Autodesk Inventor part; units mm, degrees
ref_plane "YZ Plane" through (0, 0, 0) normal (1, 0, 0) x (0, 1, 0)
ref_plane "XZ Plane" through (0, 0, 0) normal (0, 1, 0) x (-1, 0, 0)
ref_plane "XY Plane" through (0, 0, 0) normal (0, 0, 1) x (1, 0, 0)
sketch "Sketch1" plane through (0, 0, 0) normal (1, 0, 0) x (0, 1, 0)
  line L0 (0, 0) -> (12.7, 0)
  line L1 (12.7, 0) -> (12.7, -25.4)
  line L2 (12.7, -25.4) -> (0, -25.4)
  line L3 (0, -25.4) -> (0, 0)
  dimension "d0" = 12.7
  dimension "d1" = 25.4
extrude "Extrusion1" add sketch "Sketch1" along normal blind 4.7752
sketch "Sketch2" plane through (0, 12.7, 0) normal (0, 1, 0) x (1, 0, 0)
  line L0 (0, 25.4) -> (4.7752, 25.4)
  line L1 (0, 0) -> (4.7752, 0)
  point P0 (2.2104, 5.08)
  point P1 (2.2104, 20.32)
  dimension "d22" = 5.08
  dimension "d23" = 5.08
hole "Hole1" at (2.2104, 12.7, -5.08) at (2.2104, 12.7, -20.32) direction (0, -1, 0) diameter 3.429 end through all
sketch "Sketch3" plane through (0, 0, 0) normal (-1, 0, 0) x (0, 0, 1)
  line L0 (0, 12.7) -> (-25.4, 12.7)
  line L1 (-25.4, 0) -> (0, 0)
  line L2 (0, 0) -> (0, 12.7)
  point P0 (-12.7, 6.35)
  dimension "d11" = 12.7
  dimension "d12" = 25.4
  dimension "d13" = 6.35
  dimension "d14" = 12.7
hole "Hole2" at (0, 6.35, -12.7) direction (1, 0, 0) diameter 3.429 end through all
properties part number "WheelIntakeSpringStop"
Design review of the part built by this model. Coordinates are the model's own, in mm. Give positions to 0.01 mm unless a question says otherwise; leave off trailing zeros. Write each loop counter-clockwise with the first axis right and the second up, starting at its lowest first coordinate (ties: lowest second). Pieces come first, ordered by that corner, then holes. Notation, with made-up numbers: M -26,87 L -22,87 A18 ccw -22,103 Z; hole C -15,78.25 d5. An arc over 180 degrees is marked long. Answer as a JSON object with one key per item and string values. Group by question number.
1) We need section C-C (y = 11.75). Give the boundary of the cut face in (x, z), and give its area (3 significant figures).
2) We need section B-B (z = -12.7). Give the boundary of the cut face in (x, y).
3) For line 1 along Z through (x, y) = (2.1, 10); line 2 along Z through (x, y) = (2.35, 6.35); line 3 along X through (y, z) = (8, -20.32), list the stretches that pass through material, from the lowest coordinate up.
4) Clearance check with flat-ended pins moving along their axes: pin 1 Ø2.5 at (y, z) = (6.35, -12.7) entering from +X; pin 2 Ø1.5 at (x, y) = (1, 1.5) entering from +Z. State where each tip first meets the part, or that it passes through.
5) We need section A-A (y = 6.35). Give the boundary of the cut face in (x, z), and give its area (3 significant figures).
6) We need section D-D (z = -20.32). Give the boundary of the cut face in (x, y).
7) Mouldability with a two-part tool opening along Z and no side actions: class faces 1 (the face through (2, 12.7, -13)), 2 (the face through (2.421, 5.835, -11.065)), 3 (the face through (2, 6, -25.4)) as released by +Z, released by -Z, zero draft, split by the parting line, or undercut.
Answer key:
{
 "1": {"outline": "M 0,-25.4 L 4.78,-25.4 L 4.78,0 L 0,0 Z; hole C 2.21,-20.32 d3.43; hole C 2.21,-5.08 d3.43", "area": "103 mm²"},
 "2": {"outline": "M 0,0 L 4.78,0 L 4.78,4.64 L 0,4.64 Z; M 0,8.06 L 4.78,8.06 L 4.78,12.7 L 0,12.7 Z"},
 "3": {"line 1": "z = -25.4 to -22.03, -18.61 to -6.79, -3.37 to 0", "line 2": "z = -25.4 to -22.03, -18.61 to -14.41, -10.99 to -6.79, -3.37 to 0", "line 3": "x = 0 to 0.5, 3.92 to 4.78"},
 "4": {"pin 1": "passes through", "pin 2": "stops at z = 0"},
 "5": {"outline": "M 0,-25.4 L 4.78,-25.4 L 4.78,-14.41 L 0,-14.41 Z; M 0,-10.99 L 4.78,-10.99 L 4.78,0 L 0,0 Z; hole C 2.21,-20.32 d3.43; hole C 2.21,-5.08 d3.43", "area": "86.4 mm²"},
 "6": {"outline": "M 0,0 L 0.5,0 L 0.5,12.7 L 0,12.7 Z; M 3.92,0 L 4.78,0 L 4.78,12.7 L 3.92,12.7 Z"},
 "7": {"face 1": "zero draft", "face 2": "undercut", "face 3": "released by -Z"}
}
